from build123d import *

# Parameters (mm, degrees)
SKETCH1_R           = 45
BOSS_EXTRUDE1_DEPTH = 26
SKETCH2_R           = 4
BOSS_EXTRUDE2_DEPTH = 4
CUT_EXTRUDE2_DEPTH  = 69.745908969
CUT_EXTRUDE4_DEPTH  = 22


with BuildPart() as part:
    # Sketch1 → Boss-Extrude1 (new body)
    with BuildSketch(Plane(origin=(0, 0, 0), x_dir=(1, 0, 0), z_dir=(0, 1, 0))):
        with Locations(Location((0, 0, 0), (0, 0, 90))):
            Circle(SKETCH1_R)
    extrude(amount=BOSS_EXTRUDE1_DEPTH)

    # Sketch2 → Boss-Extrude2 (add)
    with BuildSketch(Plane(origin=(0, 26, 0), x_dir=(1, 0, 0), z_dir=(0, 1, 0))):
        with Locations(Location((0, 0, 0), (0, 0, 270))):
            Circle(SKETCH2_R)
    extrude(amount=BOSS_EXTRUDE2_DEPTH)

    # Sketch4 → Cut-Extrude2 (cut, through all)
    with BuildSketch(Plane(origin=(0, 26, 0), x_dir=(1, 0, 0), z_dir=(0, 1, 0))):
        with BuildLine():
            Line((-1.818379611, 7.790603031), (-7, 34))
            Line((-7, 34), (0, 42))
            Line((0, 42), (7, 34))
            Line((7, 34), (1.818379611, 7.790603031))
            ThreePointArc((1.818379611, 7.790603031), (0, 8), (-1.818379611, 7.790603031))
        make_face()
        with BuildLine():
            Line((4.222999679, 6.794576787), (19.091883092, 28.991378029))
            Line((19.091883092, 28.991378029), (29.69848481, 29.69848481))
            Line((29.69848481, 29.69848481), (28.991378029, 19.091883092))
            Line((28.991378029, 19.091883092), (6.794576787, 4.222999679))
            ThreePointArc((6.794576787, 4.222999679), (5.656854249, 5.656854249), (4.222999679, 6.794576787))
        make_face()
        with BuildLine():
            Line((7.790603031, 1.818379611), (34, 7))
            Line((34, 7), (42, 0))
            Line((42, 0), (34, -7))
            Line((34, -7), (7.790603031, -1.818379611))
            ThreePointArc((7.790603031, -1.818379611), (8, 0), (7.790603031, 1.818379611))
        make_face()
        with BuildLine():
            Line((6.794576787, -4.222999679), (28.991378029, -19.091883092))
            Line((28.991378029, -19.091883092), (29.69848481, -29.69848481))
            Line((29.69848481, -29.69848481), (19.091883092, -28.991378029))
            Line((19.091883092, -28.991378029), (4.222999679, -6.794576787))
            ThreePointArc((4.222999679, -6.794576787), (5.656854249, -5.656854249), (6.794576787, -4.222999679))
        make_face()
        with BuildLine():
            Line((1.818379611, -7.790603031), (7, -34))
            Line((7, -34), (0, -42))
            Line((0, -42), (-7, -34))
            Line((-7, -34), (-1.818379611, -7.790603031))
            ThreePointArc((-1.818379611, -7.790603031), (0, -8), (1.818379611, -7.790603031))
        make_face()
        with BuildLine():
            Line((-4.222999679, -6.794576787), (-19.091883092, -28.991378029))
            Line((-19.091883092, -28.991378029), (-29.69848481, -29.69848481))
            Line((-29.69848481, -29.69848481), (-28.991378029, -19.091883092))
            Line((-28.991378029, -19.091883092), (-6.794576787, -4.222999679))
            ThreePointArc((-6.794576787, -4.222999679), (-5.656854249, -5.656854249), (-4.222999679, -6.794576787))
        make_face()
        with BuildLine():
            Line((-7.790603031, -1.818379611), (-34, -7))
            Line((-34, -7), (-42, 0))
            Line((-42, 0), (-34, 7))
            Line((-34, 7), (-7.790603031, 1.818379611))
            ThreePointArc((-7.790603031, 1.818379611), (-8, 0), (-7.790603031, -1.818379611))
        make_face()
        with BuildLine():
            Line((-6.794576787, 4.222999679), (-28.991378029, 19.091883092))
            Line((-28.991378029, 19.091883092), (-29.69848481, 29.69848481))
            Line((-29.69848481, 29.69848481), (-19.091883092, 28.991378029))
            Line((-19.091883092, 28.991378029), (-4.222999679, 6.794576787))
            ThreePointArc((-4.222999679, 6.794576787), (-5.656854249, 5.656854249), (-6.794576787, 4.222999679))
        make_face()
    extrude(amount=-CUT_EXTRUDE2_DEPTH, mode=Mode.SUBTRACT)

    # Sketch6 → Cut-Revolve4 (revolve, cut)
    with BuildSketch(Plane(origin=(0, 0, 0), x_dir=(0, 0, -1), z_dir=(1, 0, 0)), mode=Mode.PRIVATE) as cut_revolve4_sk:
        Polygon((-45, 20.5), (-43, 19), (-43, 13), (-43, 7), (-45, 5.5), align=None)
    revolve(cut_revolve4_sk.sketch.rotate(Axis((0, 0, 0), (0, 1, 0)), 180), axis=Axis((0, 0, 0), (0, 1, 0)), mode=Mode.SUBTRACT)

    # Sketch9 → Cut-Extrude4 (cut)
    with BuildSketch(Plane(origin=(0, 30, 0), x_dir=(1, 0, 0), z_dir=(0, 1, 0))):
        with BuildLine():
            Line((-1.939071943, 1.95), (1.939071943, 1.95))
            ThreePointArc((1.939071943, 1.95), (0, -2.75), (-1.939071943, 1.95))
        make_face()
    extrude(amount=-CUT_EXTRUDE4_DEPTH, mode=Mode.SUBTRACT)


solid = part.part
Here's how the part is built. I have some questions about the finished solid (model axes, mm). A direction names the side the tool comes from. Round coordinates to 2 decimals unless told otherwise and drop trailing zeros. Write each loop counter-clockwise with the first axis right and the second up, starting at its lowest first coordinate (ties: lowest second). Pieces come first, ordered by that corner, then holes.
1. I need wall thicknesses on L1, parallel to X at y = 22, z = 0; L2, parallel to X at y = 14, z = 0; L3, parallel to Y at x = -10, z = 15.5. Which ranges of each line are inside material? Lowest first, please.
2. Will these pins go through, and if not, where does the flat tip stop? pin 1 Ø3 at (y, z) = (26.5, 5.5) entering from -X; pin 2 Ø12 at (y, z) = (20, -32.5) entering from -X; pin 3 Ø1.4 at (x, z) = (0, 0) entering from +Y.
3. Suppose I cut it at B-B (y = 2). State how many separate pieces and enclosed holes the cut face has, and give its area (3 significant figures).
4. If we mould it in two halves opening along X, with no side actions, what happens to faces 1 (the cylindrical face through (17.235, 2.712, -41.569)), 2 (the cylindrical face through (-8, 13, 0)), 3 (the flat face through (-1, 0, 1))? For each: released by +X, released by -X, zero draft, split by the parting line, or undercut.
5. Suppose I cut it at A-A (y = 28). List the corners of the cut face in (x, z) for me.
6. For faces 4 (the flat face through (0, 30, -3)), 5 (the flat face through (29.35, 13.18, -24.47)), 6 (the cylindrical face through (-42.634, 13.084, 5.598)), which set-ups out of +Z, -Z, +X, -X, +Y, -Y let a thin tool reach every point of the face, with its end or its side?
Answer sheet:
1. L1: x = -45 to -42, -8 to -2.75, 2.75 to 8, 42 to 45
1. L2: x = -43 to -42, -8 to -2.75, 2.75 to 8, 42 to 43
1. L3: y = 0 to 26
2. pin 1: stops at x = -44.81
2. pin 2: stops at x = -36.35
2. pin 3: stops at y = 8
3. separate pieces: 1
3. enclosed holes: 8
3. area: 4,070 mm2
4. face 1: split by the parting line
4. face 2: undercut
4. face 3: zero draft
5. outline: circle Ø8 at (0, 0); hole (-1.94, -1.95) - (1.94, -1.95) arc R2.75 ccw (long way) to start
6. face 4: +Z, -Z, +X, -X, +Y
6. face 5: +Y, -Y
6. face 6: none
